Read the model definition and answer for the solid it produces. Units are mm, in the model's axes. A direction names the side the tool comes from. Round coordinates to 2 decimals unless told otherwise and drop trailing zeros. Write each loop counter-clockwise with the first axis right and the second up, starting at its lowest first coordinate (ties: lowest second). Pieces come first, ordered by that corner, then holes. Notation, with made-up numbers: (-7.5, 1) -> (24.5, 1) arc R24 cw to (24.5, 36) -> close; hole circle Ø7 at (-20.5, -17). An arc over 180 degrees is marked (long way). Return JSON: item names as keys, results as strings.
from build123d import *

# Parameters (mm, degrees)
F0_R     = 22.5
F1_DEPTH = 5
F2_R     = 13.05
F3_DEPTH = 29
F4_R     = 4
F5_DEPTH = 44
F6_SIZE  = 1


# Not quite as in the source:
# - a feature names something its author has since deleted; it is built from what else it names


with BuildPart() as f1:
    # F0 (on Top) → F1 (new body)
    with BuildSketch(Plane.XY):
        Circle(F0_R)
    extrude(amount=F1_DEPTH)

    # F2 (on Top) → F3 (join)
    with BuildSketch(Plane.XY):
        Circle(F2_R)
    extrude(amount=F3_DEPTH)

    # F4 (on Top) → F5 (join)
    with BuildSketch(Plane.XY):
        Circle(F4_R)
    extrude(amount=F5_DEPTH)

    # F6
    f6_edges = [f1.edges().sort_by_distance(p)[0] for p in [
        (-22.5, 0, 0),
        (-13.05, 0, 29),
        (-4, 0, 44),
    ]]
    chamfer(f6_edges, length=F6_SIZE)


solid = f1.part
Item 1: Section A-A (x = 0) is taken. Give the vertices of the cut face in (y, z), then the cut area to 3 significant figures.
Worked answers:
{"outline": "(-22.5, 1) -> (-21.5, 0) -> (21.5, 0) -> (22.5, 1) -> (22.5, 5) -> (13.05, 5) -> (13.05, 28) -> (12.05, 29) -> (4, 29) -> (4, 43) -> (3, 44) -> (-3, 44) -> (-4, 43) -> (-4, 29) -> (-12.05, 29) -> (-13.05, 28) -> (-13.05, 5) -> (-22.5, 5) -> close", "area": "968 mm2"}
Item 2: Section C-C (z = 39.5) is taken. Give the vertices of the cut face in (x, y).
Worked answers:
{"outline": "circle Ø8 at (0, 0)"}
Item 3: Flat-ended cylindrical pins translate along their axes: pin 1 (5 mm diameter, centred on x = 4.5, z = 20, fed in from -Y); pin 2 (5 mm diameter, centred on x = -8.5, y = 16.5, fed in from +Z); pin 3 (8 mm diameter, centred on x = -6, z = 33.5, fed in from +Y). Find the tip coordinate at first contact, or state that the pin passes through.
Worked answers:
{"pin 1": "stops at y = -12.9", "pin 2": "stops at z = 5", "pin 3": "stops at y = 3.46"}
Item 4: A tool of negligible diameter and unlimited length cuts with its end or side. For faces 1 (the flat face through (0, 0, 44)), 2 (the cylindrical face through (-9.62, 8.82, 16.34)), from which of +Z, -Z, +X, -X, +Y, -Y can it reach the whole face along a straight path? Write none if from no direction.
Worked answers:
{"face 1": "+Z, +X, -X, +Y, -Y", "face 2": "+Z"}
Item 5: Straight lines are drawn through the part: L1, parallel to Z at x = -6.5, y = 13; L2, parallel to Z at x = 2, y = 10.5; L3, parallel to X at y = 0, z = 14.5. For each, find the intervals that lie inside material, in ascending order. Write a range as [from, to].
Worked answers:
{"L1": "z = [0, 5]", "L2": "z = [0, 29]", "L3": "x = [-13.05, 13.05]"}
Item 6: Section D-D (z = 22.5) is taken. Give the vertices of the cut face in (x, y), then the cut area to 3 significant figures.
Worked answers:
{"outline": "circle Ø26.1 at (0, 0)", "area": "535 mm2"}
